Build history of the part. All positions in model axes, mm. Give positions to 0.01 mm unless a question says otherwise; leave off trailing zeros. Order: outer loops, then holes, each group sorted by start corner. A loop starts at its lowest first (then second) coordinate and runs counter-clockwise, first axis right, second up. Notation, with made-up numbers: (49, 26.25) - (86, 26.25) arc R20 cw to (86, 47.25) - close; hole circle Ø6 at (-4.5, 59.25). An arc over 180 degrees is marked (long way). Write each question's results on one line, items separated by ' | '. Start each with the question number.
1) Drop flat-ended pins along their axis: pin 1 Ø1.9 at (y, z) = (3.5, -26.5) entering from +X; pin 2 Ø3 at (y, z) = (4, -19) entering from -X. Give the stop position or say it passes through.
2) Cut at A-A on z = -25. List the corners of the cut face in (x, y), plus the area to 3 significant figures.
3) Cut at C-C on x = 63. List the corners of the cut face in (y, z), plus the area to 3 significant figures.
4) Cut at B-B on y = 3.25. State how many separate pieces and enclosed holes the cut face has, plus the area to 3 significant figures.
5) Drill centre lines: line 1 along Z through (x, y) = (32, 5); line 2 along Z through (x, y) = (12, 5); line 3 along X through (y, z) = (3, -18). Where is each one in solid material? Low to high. Write a range as from..to.
from build123d import *

# Parameters (mm, degrees)
SKETCH1_W           = 140
SKETCH1_H           = 60
BOSS_EXTRUDE1_DEPTH = 6.35
SKETCH3_R           = 14.295
SKETCH3_R_2         = 2.75
CUT_EXTRUDE2_DEPTH  = 7.35
CUT_EXTRUDE3_REACH  = 8.35
SKETCH4_R           = 2.75
SKETCH4_W           = 20
SKETCH4_H           = 40


with BuildPart() as part:
    # Sketch1 → Boss-Extrude1 (new body)
    with BuildSketch(Plane(origin=(0, 0, 0), x_dir=(1, 0, 0), z_dir=(0, 1, 0))):
        with Locations((11.204600864, 33.763107794)):
            Rectangle(SKETCH1_W, SKETCH1_H)
    extrude(amount=BOSS_EXTRUDE1_DEPTH)

    # Sketch3 → Cut-Extrude2 (cut, through all)
    with BuildSketch(Plane(origin=(0, 6.35, 0), x_dir=(1, 0, 0), z_dir=(0, 1, 0))):
        with Locations((21.204600864, 33.763107794)):
            Circle(SKETCH3_R)
        with Locations((30.924600864, 10.296501734)):
            Circle(SKETCH3_R_2)
        with Locations((11.484600864, 10.296501734)):
            Circle(SKETCH3_R_2)
        with Locations((11.484600864, 57.229713855)):
            Circle(SKETCH3_R_2)
        with Locations((30.924600864, 57.229713855)):
            Circle(SKETCH3_R_2)
    extrude(amount=-CUT_EXTRUDE2_DEPTH, mode=Mode.SUBTRACT)

    # Sketch4 → Cut-Extrude3 (cut, up to next)
    with BuildSketch(Plane(origin=(0, 6.35, 0), x_dir=(1, 0, 0), z_dir=(0, 1, 0)), mode=Mode.PRIVATE) as cut_extrude3_sk1:
        with Locations((71.204600864, 53.763107794)):
            Circle(SKETCH4_R)
    cut_extrude3_tool1 = extrude(cut_extrude3_sk1.sketch, amount=-CUT_EXTRUDE3_REACH, mode=Mode.PRIVATE) & part.part
    add(cut_extrude3_tool1.solids().sort_by_distance((71.204601, 6.35, -53.763108))[0], mode=Mode.SUBTRACT)
    # Sketch4 → Cut-Extrude3 (cut, up to next)
    with BuildSketch(Plane(origin=(0, 6.35, 0), x_dir=(1, 0, 0), z_dir=(0, 1, 0)), mode=Mode.PRIVATE) as cut_extrude3_sk2:
        with Locations((-48.795399136, 53.763107794)):
            Circle(SKETCH4_R)
    cut_extrude3_tool2 = extrude(cut_extrude3_sk2.sketch, amount=-CUT_EXTRUDE3_REACH, mode=Mode.PRIVATE) & part.part
    add(cut_extrude3_tool2.solids().sort_by_distance((-48.795399, 6.35, -53.763108))[0], mode=Mode.SUBTRACT)
    # Sketch4 → Cut-Extrude3 (cut, up to next)
    with BuildSketch(Plane(origin=(0, 6.35, 0), x_dir=(1, 0, 0), z_dir=(0, 1, 0)), mode=Mode.PRIVATE) as cut_extrude3_sk3:
        with Locations((-28.795399136, 13.763107794)):
            Circle(SKETCH4_R)
    cut_extrude3_tool3 = extrude(cut_extrude3_sk3.sketch, amount=-CUT_EXTRUDE3_REACH, mode=Mode.PRIVATE) & part.part
    add(cut_extrude3_tool3.solids().sort_by_distance((-28.795399, 6.35, -13.763108))[0], mode=Mode.SUBTRACT)
    # Sketch4 → Cut-Extrude3 (cut, up to next)
    with BuildSketch(Plane(origin=(0, 6.35, 0), x_dir=(1, 0, 0), z_dir=(0, 1, 0)), mode=Mode.PRIVATE) as cut_extrude3_sk4:
        with Locations((71.204600864, 23.763107794)):
            Rectangle(SKETCH4_W, SKETCH4_H)
    cut_extrude3_tool4 = extrude(cut_extrude3_sk4.sketch, amount=-CUT_EXTRUDE3_REACH, mode=Mode.PRIVATE) & part.part
    add(cut_extrude3_tool4.solids().sort_by_distance((71.204601, 6.35, -23.763108))[0], mode=Mode.SUBTRACT)
    # Sketch4 → Cut-Extrude3 (cut, up to next)
    with BuildSketch(Plane(origin=(0, 6.35, 0), x_dir=(1, 0, 0), z_dir=(0, 1, 0)), mode=Mode.PRIVATE) as cut_extrude3_sk5:
        with Locations((-48.795399136, 23.763107794)):
            Rectangle(SKETCH4_W, SKETCH4_H)
    cut_extrude3_tool5 = extrude(cut_extrude3_sk5.sketch, amount=-CUT_EXTRUDE3_REACH, mode=Mode.PRIVATE) & part.part
    add(cut_extrude3_tool5.solids().sort_by_distance((-48.795399, 6.35, -23.763108))[0], mode=Mode.SUBTRACT)


solid = part.part
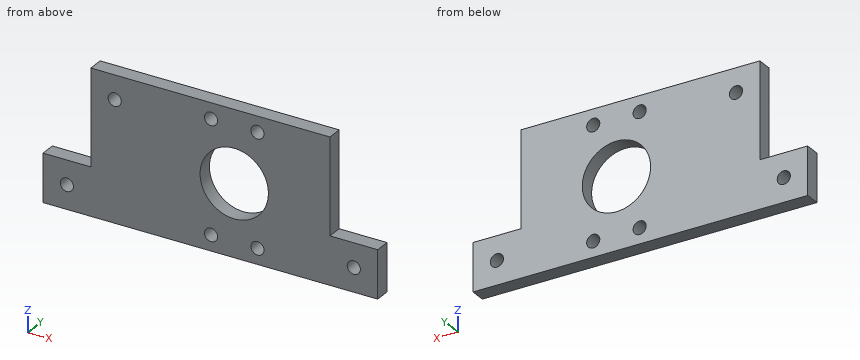
Results:
1) pin 1: x = 61.2 | pin 2: x = -38.8
2) outline: (-38.8, 0) - (9.91, 0) - (9.91, 6.35) - (-38.8, 6.35) - close; (32.5, 0) - (61.2, 0) - (61.2, 6.35) - (32.5, 6.35) - close | area: 492 mm^2
3) outline: (0, -63.76) - (6.35, -63.76) - (6.35, -43.76) - (0, -43.76) - close | area: 127 mm^2
4) separate pieces: 1 | enclosed holes: 8 | area: 5,990 mm^2
5) line 1: -63.76..-59.76, -54.7..-43.13, -24.39..-12.83, -7.77..-3.76 | line 2: -63.76..-59.93, -54.53..-44.7, -22.83..-13, -7.6..-3.76 | line 3: -38.8..61.2
